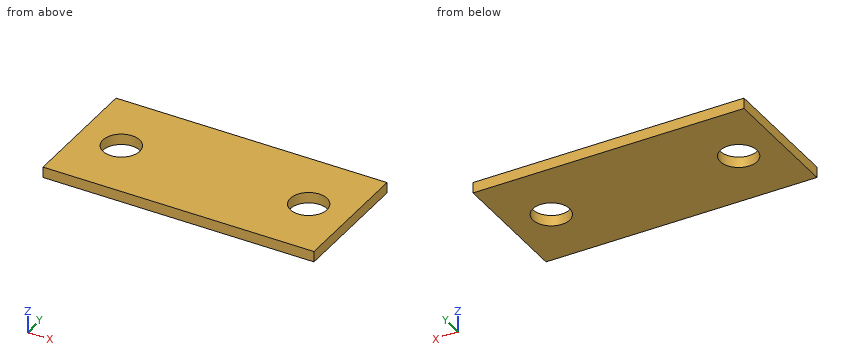
Autodesk Inventor part; units mm, degrees
ref_plane "YZ Plane" through (0, 0, 0) normal (1, 0, 0) x (0, 1, 0)
ref_plane "XZ Plane" through (0, 0, 0) normal (0, 1, 0) x (-1, 0, 0)
ref_plane "XY Plane" through (0, 0, 0) normal (0, 0, 1) x (1, 0, 0)
sketch "Sketch1" plane through (0, 0, 0) normal (0, 0, 1) x (1, 0, 0)
  line L0 (-20.25, -9.5) -> (20.25, -9.5)
  line L1 (20.25, -9.5) -> (20.25, 9.5)
  line L2 (20.25, 9.5) -> (-20.25, 9.5)
  line L3 (-20.25, 9.5) -> (-20.25, -9.5)
  line L4 (-20.25, -9.5) -> (20.25, 9.5) construction
  line L5 (20.25, -9.5) -> (-20.25, 9.5) construction
  point P0 (0, 0)
  dimension "d0" = 40.5
  dimension "d1" = 19
extrude "Extrusion1" add sketch "Sketch1" along normal blind 1.6
sketch "Sketch2" plane through (0, 0, 1.6) normal (0, 0, 1) x (1, 0, 0)
  line L0 (-14, 0) -> (14, 0) construction
  point P0 (0, 0)
  point P1 (0, 0)
  dimension "d4" = 28
hole "Hole1" at (-14, 0, 1.6) at (14, 0, 1.6) direction (0, 0, -1) diameter 5.5 depth 8 tip angle 118
properties part number "Platine_Gleichrichter"
Here's how the part is built. I have some questions about the finished solid (model axes, mm). Coordinates: 2 decimals unless noted, no trailing zeros. Order: outer loops, then holes, each group sorted by start corner. A loop starts at its lowest first (then second) coordinate and runs counter-clockwise, first axis right, second up.
1) I need wall thicknesses on line 1 (X direction, y = 0, z = 1.05); line 2 (X direction, y = 1.5, z = 0.15); line 3 (Y direction, x = 14, z = 1.2). Which ranges of each line are inside material? Lowest first, please.
2) Imagine slicing it at A-A on x = 14. List the corners of the cut face in (y, z) for me, and give its area (3 significant figures).
3) Imagine slicing it at D-D on x = -15.5. List the corners of the cut face in (y, z) for me, and give its area (3 significant figures).
4) Imagine slicing it at B-B on y = 0. List the corners of the cut face in (x, z) for me.
5) Imagine slicing it at C-C on z = 0.6. List the corners of the cut face in (x, y) for me.
Response values:
1. line 1: x = -20.25 to -16.75, -11.25 to 11.25, 16.75 to 20.25
1. line 2: x = -20.25 to -16.3, -11.7 to 11.7, 16.3 to 20.25
1. line 3: y = -9.5 to -2.75, 2.75 to 9.5
2. outline: (-9.5, 0) - (-2.75, 0) - (-2.75, 1.6) - (-9.5, 1.6) - close; (2.75, 0) - (9.5, 0) - (9.5, 1.6) - (2.75, 1.6) - close
2. area: 21.6 mm2
3. outline: (-9.5, 0) - (-2.3, 0) - (-2.3, 1.6) - (-9.5, 1.6) - close; (2.3, 0) - (9.5, 0) - (9.5, 1.6) - (2.3, 1.6) - close
3. area: 23.0 mm2
4. outline: (-20.25, 0) - (-16.75, 0) - (-16.75, 1.6) - (-20.25, 1.6) - close; (-11.25, 0) - (11.25, 0) - (11.25, 1.6) - (-11.25, 1.6) - close; (16.75, 0) - (20.25, 0) - (20.25, 1.6) - (16.75, 1.6) - close
5. outline: (-20.25, -9.5) - (20.25, -9.5) - (20.25, 9.5) - (-20.25, 9.5) - close; hole circle Ø5.5 at (-14, 0); hole circle Ø5.5 at (14, 0)
